Check sheet for the modelled part. Datum: model origin and axes. Units: mm. A direction names the side the tool comes from. Give positions to 0.01 mm unless a question says otherwise; leave off trailing zeros. Write each loop counter-clockwise with the first axis right and the second up, starting at its lowest first coordinate (ties: lowest second). Pieces come first, ordered by that corner, then holes. Notation, with made-up numbers: (13.25, -9) -> (36.25, -9) arc R31 ccw to (36.25, 19) -> close; hole circle Ø8 at (17, -31). An arc over 180 degrees is marked (long way). Use a Markdown table: item, result. Add a question column.
1. Cross-section at A-A (y = 0.35). Enter the section's corners in (x, z), then the cut area to 3 significant figures.
2. Cross-section at D-D (z = -7.75). Enter the section's corners in (x, y), then the cut area to 3 significant figures.
3. Gauge pin test, flat end, axial feed: P1, Ø1, axis at x = 3, z = -12, coming from the +Y side. Record the tip position at first contact, or that the pin passes through.
4. Release check for a two-part mould opening along Z. For faces 1 (the flat face through (1.295, 0.4, -12.2)), 2 (the flat face through (0.687, 0.413, -9.495)), 3 (the flat face through (3, 0.787, -12)) record: released by +Z, released by -Z, zero draft, split by the parting line, or undercut.
5. Cross-section at C-C (z = -6). Enter the section's corners in (x, y), then the cut area to 3 significant figures.
6. Scan lines: probe 1 along Y at (x, z) = (3.5, -5.75); probe 2 along Y at (x, z) = (10.5, -5.25); probe 3 along X at (y, z) = (0.55, -13.5). Record each from-to range of solid material in increasing order. Write a range as [from, to].
7. Cross-section at B-B (z = -3.25). Enter the section's corners in (x, y).
8. Set-up check for faces 4 (the flat face through (0, 0.4, -3.1)), 5 (the flat face through (0.39, 0.42, -5.84)), 6 (the flat face through (5.4, 0.787, -12.6)): record each of +Z, -Z, +X, -X, +Y, -Y from which the full face is reachable in a straight line by a thin tool's end or side.
from build123d import *

# Parameters (mm, degrees)
BOSS_EXTRUDE1_DEPTH = 9.753600003
SKETCH2_W           = 8.686799997
SKETCH2_H           = 0.8382
BOSS_EXTRUDE2_DEPTH = 1.295399997
BOSS_EXTRUDE3_DEPTH = 0.2032
SKETCH4_W           = 0.762
SKETCH4_H           = 2.032
CUT_EXTRUDE1_DEPTH  = 19.680648463
SKETCH5_W           = 8.382
SKETCH5_H           = 5.6388
BOSS_EXTRUDE4_DEPTH = 0.0762
SKETCH6_W           = 0.889000002
SKETCH6_H           = 3.048
CUT_EXTRUDE2_DEPTH  = 0.0508
SKETCH7_W           = 0.889
SKETCH7_H           = 3.048
CUT_EXTRUDE3_DEPTH  = 0.0508
SKETCH8_W           = 0.889
SKETCH8_H           = 3.048
CUT_EXTRUDE4_DEPTH  = 0.0508
SKETCH9_W           = 0.889
SKETCH9_H           = 3.048
CUT_EXTRUDE5_DEPTH  = 0.0508
SKETCH10_W          = 0.889
SKETCH10_H          = 3.048
CUT_EXTRUDE6_DEPTH  = 0.0508
SKETCH11_W          = 0.888999999
SKETCH11_H          = 3.301999998
CUT_EXTRUDE7_DEPTH  = 0.0508
SKETCH12_W          = 0.888999999
SKETCH12_H          = 3.301999998
CUT_EXTRUDE8_DEPTH  = 0.0508
SKETCH13_W          = 0.889
SKETCH13_H          = 3.048
CUT_EXTRUDE9_DEPTH  = 0.0508
DRAFT1_ANGLE        = 49.398705355
DRAFT2_ANGLE        = 49.635463485
FILLET2_R           = 0.050800005
FILLET3_R           = 0.254
FILLET4_R           = 0.762


with BuildPart() as part:
    # Sketch1 → Boss-Extrude1 (new body)
    with BuildSketch(Plane(origin=(1.2954, 0, 0), x_dir=(0, -1, 0), z_dir=(-1, 0, 0))):
        Polygon((-0.8382, 0), (-0.8382, -14.391699969), (-0.5842, -15.026699969), (0, -15.026699969), (0, 0), align=None)
    extrude(amount=-BOSS_EXTRUDE1_DEPTH)

    # Sketch2 → Boss-Extrude2 (add)
    with BuildSketch(Plane.ZY.offset(-1.2954)):
        with Locations((-4.343399999, 0.4191)):
            Rectangle(SKETCH2_W, SKETCH2_H)
    extrude(amount=BOSS_EXTRUDE2_DEPTH)

    # Sketch3 → Boss-Extrude3 (add)
    with BuildSketch(Plane.XZ):
        with BuildLine():
            Line((0, -0.762000007), (0, 0))
            Line((0, 0), (11.049, 0))
            Line((11.049, 0), (11.049, -0.762000007))
            ThreePointArc((11.049, -0.762000007), (5.5245, -1.709233412), (0, -0.762000007))
        make_face()
    extrude(amount=BOSS_EXTRUDE3_DEPTH)

    # Sketch4 → Cut-Extrude1 (cut, through all)
    with BuildSketch(Plane(origin=(0, 0.8382, 0), x_dir=(-1, 0, 0), z_dir=(0, 1, 0))):
        with Locations((-0.381, -6.4008)):
            Rectangle(SKETCH4_W, SKETCH4_H)
    extrude(amount=-CUT_EXTRUDE1_DEPTH, mode=Mode.SUBTRACT)

    # Sketch5 → Boss-Extrude4 (add)
    with BuildSketch(Plane(origin=(0, 0.8382, 0), x_dir=(-1, 0, 0), z_dir=(0, 1, 0))):
        with Locations((-5.483604679, -3.9624)):
            Rectangle(SKETCH5_W, SKETCH5_H)
    extrude(amount=BOSS_EXTRUDE4_DEPTH)

    # Sketch6 → Cut-Extrude2 (cut)
    with BuildSketch(Plane(origin=(0, 0.8382, 0), x_dir=(-1, 0, 0), z_dir=(0, 1, 0))):
        with Locations((-1.9685, -12.496800003)):
            Rectangle(SKETCH6_W, SKETCH6_H)
    extrude(amount=-CUT_EXTRUDE2_DEPTH, mode=Mode.SUBTRACT)

    # Sketch7 → Cut-Extrude3 (cut)
    with BuildSketch(Plane(origin=(0, 0.8382, 0), x_dir=(-1, 0, 0), z_dir=(0, 1, 0))):
        with Locations((-4.254499999, -12.496800003)):
            Rectangle(SKETCH7_W, SKETCH7_H)
    extrude(amount=-CUT_EXTRUDE3_DEPTH, mode=Mode.SUBTRACT)

    # Sketch8 → Cut-Extrude4 (cut)
    with BuildSketch(Plane(origin=(0, 0.8382, 0), x_dir=(-1, 0, 0), z_dir=(0, 1, 0))):
        with Locations((-3.111499999, -12.496800003)):
            Rectangle(SKETCH8_W, SKETCH8_H)
    extrude(amount=-CUT_EXTRUDE4_DEPTH, mode=Mode.SUBTRACT)

    # Sketch9 → Cut-Extrude5 (cut)
    with BuildSketch(Plane(origin=(0, 0.8382, 0), x_dir=(-1, 0, 0), z_dir=(0, 1, 0))):
        with Locations((-9.969500001, -12.496800003)):
            Rectangle(SKETCH9_W, SKETCH9_H)
    extrude(amount=-CUT_EXTRUDE5_DEPTH, mode=Mode.SUBTRACT)

    # Sketch10 → Cut-Extrude6 (cut)
    with BuildSketch(Plane(origin=(0, 0.8382, 0), x_dir=(-1, 0, 0), z_dir=(0, 1, 0))):
        with Locations((-6.5405, -12.496800003)):
            Rectangle(SKETCH10_W, SKETCH10_H)
    extrude(amount=-CUT_EXTRUDE6_DEPTH, mode=Mode.SUBTRACT)

    # Sketch11 → Cut-Extrude7 (cut)
    with BuildSketch(Plane(origin=(0, 0.8382, 0), x_dir=(-1, 0, 0), z_dir=(0, 1, 0))):
        with Locations((-5.3975, -12.623800002)):
            Rectangle(SKETCH11_W, SKETCH11_H)
    extrude(amount=-CUT_EXTRUDE7_DEPTH, mode=Mode.SUBTRACT)

    # Sketch12 → Cut-Extrude8 (cut)
    with BuildSketch(Plane(origin=(0, 0.8382, 0), x_dir=(-1, 0, 0), z_dir=(0, 1, 0))):
        with Locations((-7.683500001, -12.623800002)):
            Rectangle(SKETCH12_W, SKETCH12_H)
    extrude(amount=-CUT_EXTRUDE8_DEPTH, mode=Mode.SUBTRACT)

    # Sketch13 → Cut-Extrude9 (cut)
    with BuildSketch(Plane(origin=(0, 0.8382, 0), x_dir=(-1, 0, 0), z_dir=(0, 1, 0))):
        with Locations((-8.826500001, -12.496800003)):
            Rectangle(SKETCH13_W, SKETCH13_H)
    extrude(amount=-CUT_EXTRUDE9_DEPTH, mode=Mode.SUBTRACT)

    # Draft1
    draft1_faces = [part.faces().sort_by_distance(p)[0] for p in [
        (0.381, 0.4191, -5.3848),
    ]]
    draft(draft1_faces, Plane(origin=(3e-09, 0, 0), x_dir=(0, 0, -1), z_dir=(-1, 0, 0)), DRAFT1_ANGLE)

    # Draft2
    draft2_faces = [part.faces().sort_by_distance(p)[0] for p in [
        (0.647700002, 0.4191, -8.686799997),
    ]]
    draft(draft2_faces, Plane(origin=(3e-09, 0, 0), x_dir=(0, 0, -1), z_dir=(-1, 0, 0)), DRAFT2_ANGLE)

    # Fillet2
    fillet2_edges = [part.edges().sort_by_distance(p)[0] for p in [
        (5.5245, 0, -1.709233412),
    ]]
    fillet(fillet2_edges, radius=FILLET2_R)

    # Fillet3
    fillet3_edges = [part.edges().sort_by_distance(p)[0] for p in [
        (3e-09, 0.4191, -8.686799997),
        (0.762, 0.4191, -7.4168),
    ]]
    fillet(fillet3_edges, radius=FILLET3_R)

    # Fillet4
    fillet4_edges = [part.edges().sort_by_distance(p)[0] for p in [
        (3e-09, 0.4191, 0),
        (11.049000003, 0.2921, -15.026699969),
        (11.049000003, 0.4191, 0),
        (1.2954, 0.2921, -15.026699969),
    ]]
    fillet(fillet4_edges, radius=FILLET4_R)


solid = part.part
Worked answers:
| question | item | result |
|---|---|---|
| 1 | outline | (0, -8.59) arc R0.25 ccw to (0.06, -8.76) -> (1.3, -10.21) -> (1.3, -14.26) arc R0.76 ccw to (2.06, -15.03) -> (10.29, -15.03) arc R0.76 ccw to (11.05, -14.26) -> (11.05, -0.76) arc R0.76 ccw to (10.29, 0) -> (0.76, 0) arc R0.76 ccw to (0, -0.76) -> (0, -5.38) -> (0.76, -6.27) -> (0.76, -7.16) arc R0.25 cw to (0.51, -7.42) -> (0, -7.42) -> close |
| 1 | area | 157 mm² |
| 2 | outline | (0, 0) -> (11.05, 0) -> (11.05, 0.84) -> (0, 0.84) -> close |
| 2 | area | 9.26 mm² |
| 3 | P1 | stops at y = 0.84 |
| 4 | face 1 | zero draft |
| 4 | face 2 | released by -Z |
| 4 | face 3 | undercut |
| 5 | outline | (0.53, 0) -> (11.05, 0) -> (11.05, 0.84) -> (9.67, 0.84) -> (9.67, 0.91) -> (1.29, 0.91) -> (1.29, 0.84) -> (0.53, 0.84) -> close |
| 5 | area | 9.46 mm² |
| 6 | probe 1 | y = [0, 0.91] |
| 6 | probe 2 | y = [0, 0.84] |
| 6 | probe 3 | x = [1.3, 11.05] |
| 7 | outline | (0, 0) -> (11.05, 0) -> (11.05, 0.84) -> (9.67, 0.84) -> (9.67, 0.91) -> (1.29, 0.91) -> (1.29, 0.84) -> (0, 0.84) -> close |
| 8 | face 4 | +Z, -Z, -X, +Y, -Y |
| 8 | face 5 | -X, +Y, -Y |
| 8 | face 6 | +Y |
